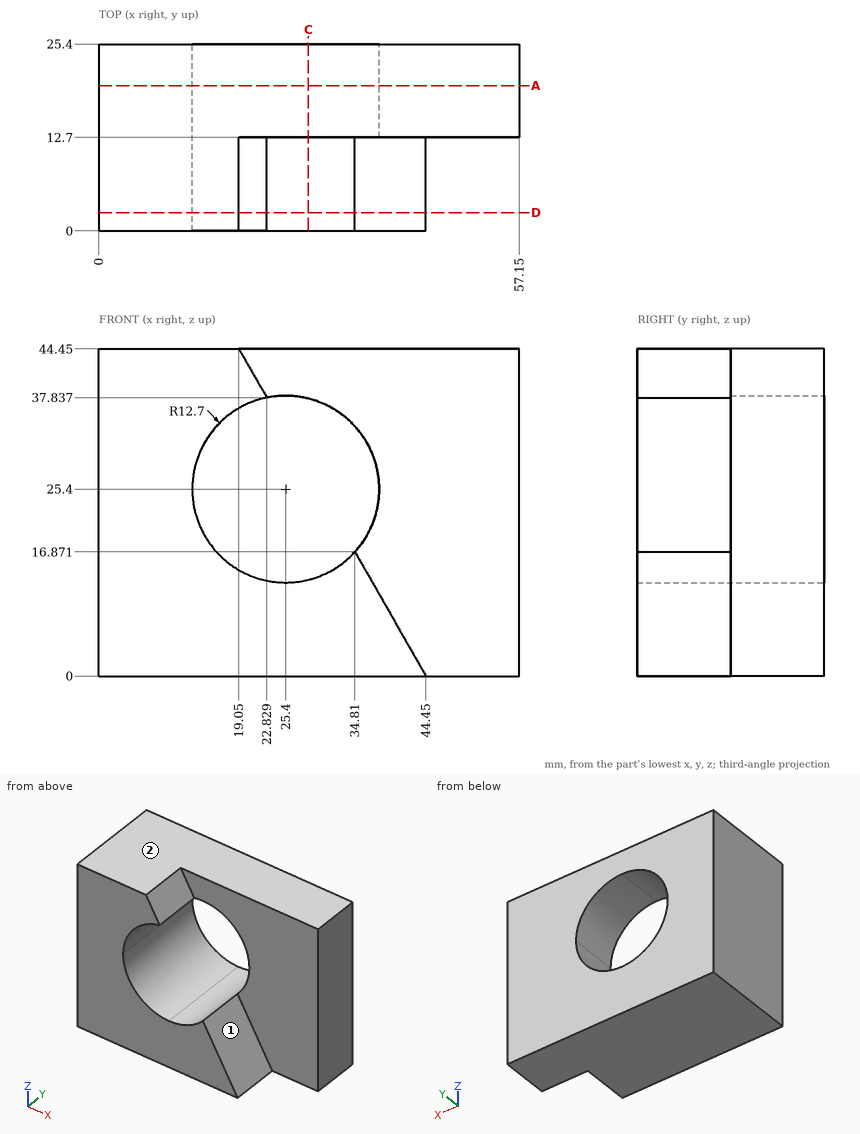
Check sheet for the drawn part. Datum: minimum x, y, z corner. Units: mm. A direction names the side the tool comes from. Round coordinates to 2 decimals unless told otherwise and drop trailing zeros. Loops run counter-clockwise (first coordinate to the right, second up) from the corner with the lowest first, then second, coordinate; pieces in that order, holes last. Notation, with made-up numbers: M 51.25,-8 L 61.25,-8 A17 ccw 61.25,-2 Z; hole C 4,77.25 d2. An arc over 180 degrees is marked long. One line per question, with ' | ' between items. Start each with the question number.
Item 1: Section check A-A (y = 19.75). Record the boundary of the cut face in (x, z).
Item 2: Section check D-D (y = 2.5). Record the boundary of the cut face in (x, z).
Item 3: Gauge pin test, flat ends, axial feed: pin 1 Ø3 at (x, y) = (38.5, 5) entering from +Z; pin 2 Ø1 at (y, z) = (10, 9) entering from +X; pin 3 Ø1 at (x, z) = (14, 22) entering from +Y; pin 4 Ø6 at (x, y) = (28.5, 11) entering from +Z. Record the tip position at first contact, or that the pin passes through.
Item 4: Section check C-C (x = 28.5). Record the boundary of the cut face in (y, z), and give its area (3 significant figures).
Item 5: Scan lines: probe 1 along Y at (x, z) = (45.5, 8); probe 2 along Z at (x, y) = (16.5, 1.25); probe 3 along X at (y, z) = (13.25, 21.5). Record each from-to range of solid material in increasing order.
Item 6: Set-up check for the marked faces 1 and 2: record each of +Z, -Z, +X, -X, +Y, -Y from which the full face is reachable in a straight line by a thin tool's end or side.
Worked out:
1) outline: M 0,0 L 57.15,0 L 57.15,44.45 L 0,44.45 Z; hole C 25.4,25.4 d25.4
2) outline: M 0,0 L 44.45,0 L 34.81,16.87 A12.7 cw long 22.83,37.84 L 19.05,44.45 L 0,44.45 Z
3) pin 1: z = 13.04 | pin 2: x = 39.59 | pin 3: through | pin 4: z = 44.45
4) outline: M 0,0 L 25.4,0 L 25.4,13.08 L 0,13.08 Z; M 12.7,37.72 L 25.4,37.72 L 25.4,44.45 L 12.7,44.45 Z | area: 418 mm^2
5) probe 1: 12.7 to 25.4 | probe 2: 0 to 16.34, 34.46 to 44.45 | probe 3: 0 to 13.31, 37.49 to 57.15
6) face 1: +Z, +X, -Y | face 2: +Z, +X, -X, +Y, -Y
